```python
from build123d import *

# Parameters (mm, degrees)
SCHIZZO2_W                   = 31
SCHIZZO2_H                   = 14
ESTRUSIONE_ESTRUSIONE1_DEPTH = 1.6
ESTRUSIONE_ESTRUSIONE2_DEPTH = 6
TAGLIO_ESTRUSIONE1_REACH     = 37.454
SCHIZZO4_R                   = 1.75


with BuildPart() as part:
    # Schizzo2 → Estrusione-Estrusione1 (new body)
    with BuildSketch(Plane(origin=(0, 0, 0), x_dir=(1, 0, 0), z_dir=(0, 1, 0))):
        with Locations((15.5, 7)):
            Rectangle(SCHIZZO2_W, SCHIZZO2_H)
    extrude(amount=ESTRUSIONE_ESTRUSIONE1_DEPTH)

    # Schizzo3 → Estrusione-Estrusione2 (add)
    with BuildSketch(Plane.ZY):
        Polygon((-14, 1.6), (-14, 11.6), (-9.5, 11.6), (-9.5, 3.6), (-4.5, 3.6), (-4.5, 11.6), (0, 11.6), (0, 1.6), align=None)
    extrude(amount=-ESTRUSIONE_ESTRUSIONE2_DEPTH)

    # Schizzo4 → Taglio-Estrusione1 (cut, up to next)
    with BuildSketch(Plane(origin=(0, 1.6, 0), x_dir=(1, 0, 0), z_dir=(0, 1, 0)), mode=Mode.PRIVATE) as taglio_estrusione1_sk1:
        with Locations(Location((24, 7, 0), (0, 0, 270))):
            Circle(SCHIZZO4_R)
    taglio_estrusione1_tool1 = extrude(taglio_estrusione1_sk1.sketch, amount=-TAGLIO_ESTRUSIONE1_REACH, mode=Mode.PRIVATE) & part.part
    add(taglio_estrusione1_tool1.solids().sort_by_distance((24, 1.6, -7))[0], mode=Mode.SUBTRACT)


solid = part.part
```
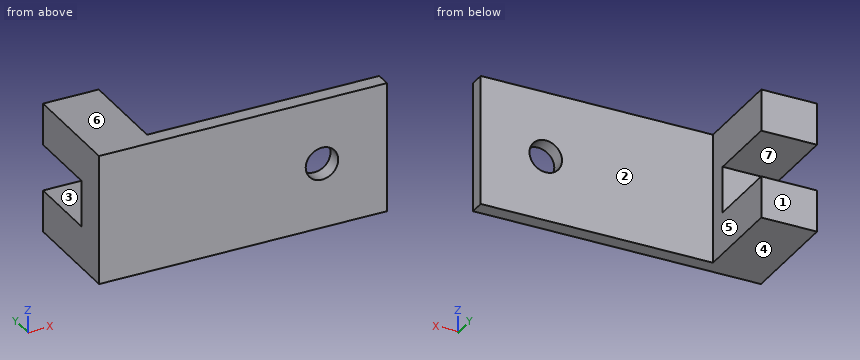
Work out the finished part from the listing and answer in its coordinate system (mm). Face numbers are marked on the shaded views. A direction names the side the tool comes from. Give positions to 0.01 mm unless a question says otherwise; leave off trailing zeros. Loops run counter-clockwise (first coordinate to the right, second up) from the corner with the lowest first, then second, coordinate; pieces in that order, holes last. Notation, with made-up numbers: M -21.5,80.5 L -8.5,80.5 A9 ccw -8.5,95.5 Z; hole C 4.25,78 d5. An arc over 180 degrees is marked long. One line per item, written item: value. Start each with the question number.
1. Determine the mould class of the marked faces 4, 5, 6 and 7 for opening direction Z: released by +Z, released by -Z, zero draft, split by the parting line, or undercut.
2. Which of the six approach directions +Z, -Z, +X, -X, +Y, -Y give full straight-line access (tool end or side, diameter ignored) to the marked faces 1, 2 and 3?
3. Find section A-A (y = 10.25). Give the vertices of the cut face in (x, z).
4. Find the intervals of material crossed by probe 1 along X at (y, z) = (1.35, -7); probe 2 along X at (y, z) = (8.5, -2.75); probe 3 along Y at (x, z) = (8.5, -4), in increasing order.
5. Find section D-D (z = -3.5). Give the vertices of the cut face in (x, y), and give its area (3 significant figures).
6. Find section B-B (z = -7). Give the vertices of the cut face in (x, y).
7. Find section C-C (x = 24). Give the vertices of the cut face in (y, z).
8. Each of these flat-tipped pins is pushed along its axis until it touches: P1, Ø1, axis at x = 10.5, z = -4, coming from the -Y side; P2, Ø1.5, axis at x = 27.5, y = 4, coming from the -Z side; P3, Ø7, axis at x = 20, z = -6, coming from the +Y side; P4, Ø4, axis at y = 6, z = -12, coming from the +X side. Where does it stop, or does it pass through?
Reported:
1. face 4: released by -Z
1. face 5: zero draft
1. face 6: released by +Z
1. face 7: undercut
2. face 1: +Z, -Z, +X, -X, +Y
2. face 2: +Z, -Z, +X, +Y
2. face 3: +X, -X, +Y
3. outline: M 0,-14 L 6,-14 L 6,-9.5 L 0,-9.5 Z; M 0,-4.5 L 6,-4.5 L 6,0 L 0,0 Z
4. probe 1: x = 0 to 22.25, 25.75 to 31
4. probe 2: x = 0 to 6
4. probe 3: y = 0 to 1.6
5. outline: M 0,0 L 31,0 L 31,1.6 L 6,1.6 L 6,11.6 L 0,11.6 Z
5. area: 110 mm²
6. outline: M 0,0 L 22.25,0 L 22.25,1.6 L 6,1.6 L 6,3.6 L 0,3.6 Z; M 25.75,0 L 31,0 L 31,1.6 L 25.75,1.6 Z
7. outline: M 0,-14 L 1.6,-14 L 1.6,-8.75 L 0,-8.75 Z; M 0,-5.25 L 1.6,-5.25 L 1.6,0 L 0,0 Z
8. P1: stops at y = 0
8. P2: passes through
8. P3: stops at y = 1.6
8. P4: stops at x = 6
